The listing builds one solid part. Answer for the finished solid, in the listing's coordinates (mm). A direction names the side the tool comes from. Coordinates: 2 decimals unless noted, no trailing zeros. Order: outer loops, then holes, each group sorted by start corner. A loop starts at its lowest first (then second) coordinate and runs counter-clockwise, first axis right, second up.
from build123d import *

# Parameters (mm, degrees)
F0_W     = 596.9
F0_H     = 1206.5
F0_W_2   = 556.9
F0_H_2   = 1166.5
F1_DEPTH = 63.5
F2_W     = 596.9
F2_H     = 1206.5
F2_R     = 107.095768
F3_DEPTH = 10
F4_R     = 5
F5_DEPTH = 596.9


with BuildPart() as f1:
    # F0 (on Front) → F1 (new body)
    with BuildSketch(Plane.XZ):
        with Locations((298.45, -603.25)):
            Rectangle(F0_W, F0_H)
        with Locations((298.45, -603.25)):
            Rectangle(F0_W_2, F0_H_2, mode=Mode.SUBTRACT)
    extrude(amount=F1_DEPTH)

    # F2 (on Front) → F3 (join)
    with BuildSketch(Plane.XZ):
        with Locations((298.45, -603.25)):
            Rectangle(F2_W, F2_H)
        with Locations((298.45, -228.6)):
            Circle(F2_R, mode=Mode.SUBTRACT)
    extrude(amount=-F3_DEPTH)

    # F4 (on Right) → F5 (cut, through all)
    with BuildSketch(Plane.YZ):
        with Locations((-30, -65)):
            Circle(F4_R)
    extrude(amount=F5_DEPTH, mode=Mode.SUBTRACT)


solid = f1.part
(1) A tool of negligible diameter and unlimited length cuts with its end or side. For faces 4 (the flat face through (20, -31, -611)), 5 (the flat face through (596.9, -27, -612)), from which of +Z, -Z, +X, -X, +Y, -Y can it reach the whole face along a straight path? Write none if from no direction.
(2) Given pin 1 Ø2 at (x, z) = (182.5, -1042) entering from -Y, flat-ended and moving along its own axis, determine where the tip first touches the part or whether it passes through.
(3) Find section C-C on z = -228.6. Determine the outline of the cut face in (x, y), then the cut area to 3 significant figures.
(4) Find section D-D on x = 179. Determine the outline of the cut face in (y, z), then the cut area to 3 significant figures.
(5) Find section B-B on y = -46. Determine the outline of the cut face in (x, z), then the cut area to 3 significant figures.
(6) Find section A-A on x = 298.45. Determine the outline of the cut face in (y, z).
(7) The mould has two halves that part along X. Classify faces 1 (the flat face through (0, -27, -612)), 2 (the flat face through (294, 10, -595)), 3 (the flat face through (295, 0, -595)): pulls with the +X half, pulls with the -X half, needs draft (parallel to the pull), parting line crosses it, or undercut.
(8) Find the intervals of material crossed by probe 1 along X at (y, z) = (-12, -418.5); probe 2 along Z at (x, y) = (142, -5.5); probe 3 along Y at (x, z) = (589.5, -65), in increasing order.
Resolved:
1. face 4: -Y
1. face 5: +Z, -Z, +X, +Y, -Y
2. pin 1: stops at y = 0
3. outline: (0, -63.5) - (20, -63.5) - (20, 0) - (191.35, 0) - (191.35, 10) - (0, 10) - close; (405.55, 0) - (576.9, 0) - (576.9, -63.5) - (596.9, -63.5) - (596.9, 10) - (405.55, 10) - close
3. area: 6,370 mm2
4. outline: (-63.5, -1206.5) - (10, -1206.5) - (10, 0) - (-63.5, 0) - (-63.5, -20) - (0, -20) - (0, -1186.5) - (-63.5, -1186.5) - close
4. area: 14,600 mm2
5. outline: (0, -1206.5) - (596.9, -1206.5) - (596.9, 0) - (0, 0) - close; hole (20, -1186.5) - (576.9, -1186.5) - (576.9, -20) - (20, -20) - close
5. area: 70,500 mm2
6. outline: (-63.5, -1206.5) - (10, -1206.5) - (10, -335.7) - (0, -335.7) - (0, -1186.5) - (-63.5, -1186.5) - close; (-63.5, -20) - (0, -20) - (0, -121.5) - (10, -121.5) - (10, 0) - (-63.5, 0) - close
7. face 1: pulls with the -X half
7. face 2: needs draft
7. face 3: undercut
8. probe 1: x = 0 to 20, 576.9 to 596.9
8. probe 2: z = -1206.5 to -1186.5, -20 to 0
8. probe 3: y = -63.5 to -35, -25 to 10
